```python
from build123d import *

# Parameters (mm, degrees)
F1_DEPTH = 63.5
F0_W     = 25.4
F0_H     = 19.05
F2_DEPTH = 25.4
F3_DEPTH = 7.366


with BuildPart() as f1:
    # F0 (on Front) → F1 (new body, symmetric)
    with BuildSketch(Plane.XZ):
        Polygon((22.225, 9.525), (-41.275, 9.525), (-41.275, -9.525), (41.275, -9.525), (41.275, 9.525), align=None)
    extrude(amount=F1_DEPTH, both=True)

    # F0 (on Front) → F2 (join, symmetric)
    with BuildSketch(Plane.XZ):
        with BuildLine():
            Line((22.225, 31.6498798487), (22.225, 9.525))
            Line((22.225, 9.525), (41.275, 9.525))
            Line((41.275, 9.525), (41.275, 31.6498798487))
            ThreePointArc((41.275, 31.6498798487), (44.5628201513, 39.5873798487), (52.5003201513, 42.8752))
            Line((52.5003201513, 42.8752), (60.325, 42.8752))
            Line((60.325, 42.8752), (60.325, 61.9252))
            Line((60.325, 61.9252), (57.422989761, 61.9252))
            add(Edge.make_bspline(
                [(47.6310352759, 61.5310624736), (50.9065534115, 61.7825559935), (54.1756772535, 61.9134758207), (57.422989761, 61.9252)],
                knots=[102.2694518038, 102.2694518038, 102.2694518038, 102.2694518038, 111.7455777331, 111.7455777331, 111.7455777331, 111.7455777331], degree=3))
            ThreePointArc((47.6310352759, 61.5310624736), (29.4350413889, 51.2607932868), (22.225, 31.6498798487))
        make_face()
        with Locations((73.025, 52.4002)):
            Rectangle(F0_W, F0_H)
    extrude(amount=F2_DEPTH, both=True)

    # F0 (on Front) → F3 (join, symmetric)
    with BuildSketch(Plane.XZ):
        with BuildLine():
            add(Edge.make_bspline(
                [(-41.275, 9.525), (-23.8146628268, 42.0589220726), (12.2805717425, 58.8168621141), (47.6310352759, 61.5310624736)],
                knots=[0, 0, 0, 0, 102.2694518038, 102.2694518038, 102.2694518038, 102.2694518038], degree=3))
            Line((-41.275, 9.525), (22.225, 9.525))
            Line((22.225, 9.525), (22.225, 31.6498798487))
            ThreePointArc((22.225, 31.6498798487), (29.4350413889, 51.2607932868), (47.6310352759, 61.5310624736))
        make_face()
    extrude(amount=F3_DEPTH, both=True)

    # F0 (on Front) → F4 (revolve)
    with BuildSketch(Plane.XZ):
        Polygon((85.725, 66.675), (85.725, 61.9252), (85.725, 42.8752), (85.725, 38.1), (111.125, 38.1), (111.125, 66.675), align=None)
    revolve(axis=Axis((85.725, 0, 52.3875), (0, 0, -1)))


solid = f1.part
```
Part model, mm, in its own coordinate system. A direction names the side the tool comes from. Round coordinates to 2 decimals unless told otherwise and drop trailing zeros. Write each loop counter-clockwise with the first axis right and the second up, starting at its lowest first coordinate (ties: lowest second). Pieces come first, ordered by that corner, then holes. Notation, with made-up numbers: (82, 59) -> (108, 59) arc R22 ccw to (108, 68) -> close; hole circle Ø1 at (86.25, 64.5). An arc over 180 degrees is marked (long way). Return JSON: item names as keys, results as strings. Group by question number.
Q1. Which spindle directions (+Z, -Z, +X, -X, +Y, -Y) get a long thin tool onto all of the face, cutting with end or side? Do faces 5 (the flat face through (60, 0, 61.925)), 6 (the cylindrical face through (29.63, 16.26, 51.49)), 7 (the cylindrical face through (29.63, -16.51, 51.49)). Say none if no direction does.
Q2. Saw through at B-B on y = 43.5. Write the cut outline in (x, z) (3 decimals).
Q3. Mould opens along X. For faces 1 (the flat face through (58, 0, 42.875)), 2 (the cylindrical face through (44.476, -0.356, 39.5)), 3 (the flat face through (-41.275, -1, 0)), 4 (the flat face through (46, -25.4, 42)) say: pulls with the +X half, pulls with the -X half, needs draft (parallel to the pull), parting line crosses it, or undercut.
Q4. Pin check, flat tips, straight feed: pin 1 (5 mm diameter, centred on x = -26, z = 31, fed in from +Y); pin 2 (10 mm diameter, centred on x = 73, y = 3.5, fed in from -Z); pin 3 (12 mm diameter, centred on y = -30.5, z = 23, fed in from -X) (3 decimals). Stop position of each tip, or through.
Q5. Probe L1, parallel to Z at x = -14, y = -22.5 (3 decimals); L2, parallel to Y at x = 9.5, z = 36.5; L3, parallel to X at y = 13.5, z = 26 (3 decimals). List the from-to ranges inside material, lowest first. Write a range as [from, to].
Q6. Saw through at C-C on z = -3. Write the cut outline in (x, y) (3 decimals), plus the area to 3 significant figures.
Q7. Saw through at A-A on x = 66. Write the cut outline in (y, z) (3 decimals), plus the area to 3 significant figures.
Answer:
{
 "1": {"face 5": "+Z, -X", "face 6": "+Z, -X, +Y", "face 7": "+Z, -X, -Y"},
 "2": {"outline": "(-41.275, -9.525) -> (41.275, -9.525) -> (41.275, 9.525) -> (-41.275, 9.525) -> close"},
 "3": {"face 1": "undercut", "face 2": "undercut", "face 3": "pulls with the -X half", "face 4": "needs draft"},
 "4": {"pin 1": "y = 7.37", "pin 2": "z = 38.1", "pin 3": "x = 22.225"},
 "5": {"L1": "[-9.525, 9.525]", "L2": "[-7.37, 7.37]", "L3": "[22.225, 41.275]"},
 "6": {"outline": "(-41.275, -63.5) -> (41.275, -63.5) -> (41.275, 63.5) -> (-41.275, 63.5) -> close", "area": "10,500 mm2"},
 "7": {"outline": "(-25.4, 42.875) -> (-16.003, 42.875) -> (-16.003, 38.1) -> (16.003, 38.1) -> (16.003, 42.875) -> (25.4, 42.875) -> (25.4, 61.925) -> (16.003, 61.925) -> (16.003, 66.675) -> (-16.003, 66.675) -> (-16.003, 61.925) -> (-25.4, 61.925) -> close", "area": "1,270 mm2"}
}
